Source: CAD feature listing. Evaluate the final solid. Frame: model axes, mm. A direction names the side the tool comes from. Round coordinates to 2 decimals unless told otherwise and drop trailing zeros. Order: outer loops, then holes, each group sorted by start corner. A loop starts at its lowest first (then second) coordinate and runs counter-clockwise, first axis right, second up.
```python
from build123d import *

# Parameters (mm, degrees)
SKETCH040_W    = 252
SKETCH040_H    = 268
PAD011_DEPTH   = 60
FILLET013_R    = 6
THICKNESS001_T = 3


with BuildPart() as part:
    # Sketch040 → Pad011 (new body)
    with BuildSketch(Plane.XY):
        with Locations((0, -134)):
            Rectangle(SKETCH040_W, SKETCH040_H)
    extrude(amount=PAD011_DEPTH)

    # Fillet013
    fillet013_edges = [part.edges().sort_by_distance(p)[0] for p in [
        (126, -268, 30),
        (-126, -268, 30),
    ]]
    fillet(fillet013_edges, radius=FILLET013_R)

    # Thickness001
    thickness001_openings = [part.faces().sort_by_distance(p)[0] for p in [
        (0, -133.969642, 60),
        (0, -133.969642, 0),
        (0, 0, 30),
    ]]
    offset(amount=THICKNESS001_T, openings=thickness001_openings)


solid = part.part
```
1. Section A-A on y = -192.5. Return loops of the section in (x, z), plus the area to 3 significant figures.
2. Access query for faces 4 (the face through (-124.289, -266.196, 30.42)), 5 (the face through (129, -133, 30)). Directions: +Z, -Z, +X, -X, +Y, -Y. A direction counts if a zero-diameter tool reaches every point of the face in a straight line with its end or side. Return the directions, or none.
3. Section B-B on z = 52.5. Return loops of the section in (x, y), plus the area to 3 significant figures.
4. Pull-direction query (X, two-part tool) for faces 1 (the face through (126.294, -268.434, 30.42)), 2 (the face through (-129, -133, 30)), 3 (the face through (124.196, -266.289, 30.42)); classes: released by +X, released by -X, zero draft, split by the parting line, or undercut.
5. First-contact query: pin 1 (12 mm diameter, centred on x = -41, z = 31, fed in from +Y). Flat tip, straight axial feed; report the tip coordinate or a pass-through.
6. Section C-C on x = -86.5. Return loops of the section in (y, z), plus the area to 3 significant figures.
7. Line query: line 1 along X through (y, z) = (-12, 7); line 2 along Y through (x, z) = (-32.5, 40.5). Output: solid intervals per line, ascending.
Result:
1. outline: (-129, 0) - (-126, 0) - (-126, 60) - (-129, 60) - close; (126, 0) - (129, 0) - (129, 60) - (126, 60) - close
1. area: 360 mm2
2. face 4: +Z, -Z, +Y
2. face 5: +Z, -Z, +X, +Y, -Y
3. outline: (-129, -262) arc R9 ccw to (-120, -271) - (120, -271) arc R9 ccw to (129, -262) - (129, 0) - (126, 0) - (126, -262) arc R6 cw to (120, -268) - (-120, -268) arc R6 cw to (-126, -262) - (-126, 0) - (-129, 0) - close
3. area: 2,360 mm2
4. face 1: released by +X
4. face 2: released by -X
4. face 3: undercut
5. pin 1: stops at y = -268
6. outline: (-271, 0) - (-268, 0) - (-268, 60) - (-271, 60) - close
6. area: 180 mm2
7. line 1: x = -129 to -126, 126 to 129
7. line 2: y = -271 to -268
